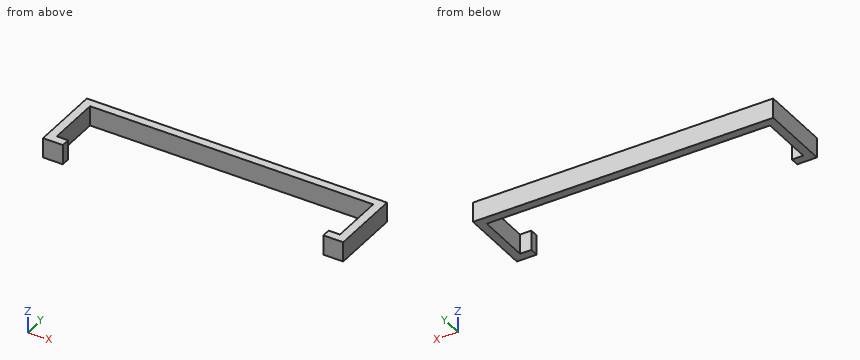
Autodesk Inventor part; units mm, degrees
ref_plane "YZ Plane" through (0, 0, 0) normal (1, 0, 0) x (0, 1, 0)
ref_plane "XZ Plane" through (0, 0, 0) normal (0, 1, 0) x (-1, 0, 0)
ref_plane "XY Plane" through (0, 0, 0) normal (0, 0, 1) x (1, 0, 0)
sketch "Szkic1" plane through (0, 0, 0) normal (0, 1, 0) x (-1, 0, 0)
  point P0 (0, 0)
sketch "Szkic2" plane through (0, 0, 0) normal (0, 1, 0) x (-1, 0, 0)
  line L0 (0, 0) -> (-100, 0)
  line L1 (-100, 0) -> (-100, 7)
  line L2 (-100, 7) -> (0, 7)
  line L3 (0, 7) -> (0, 0)
  dimension "d0" = 100
  dimension "d1" = 7
extrude "Wyciągnięcie proste1" add sketch "Szkic2" along normal blind 3
sketch "Szkic3" plane through (0, 3, 0) normal (0, 1, 0) x (1, 0, 0)
  line L0 (0, 0) -> (-3, 0)
  line L1 (-3, 0) -> (-3, -7)
  line L2 (-3, -7) -> (0, -7)
  line L3 (0, -7) -> (0, 0)
  line L4 (100, -7) -> (100, 0)
  line L5 (100, 0) -> (103, 0)
  line L6 (103, 0) -> (103, -7)
  line L7 (103, -7) -> (100, -7)
  line L8 (100, -7) -> (100, 0)
  dimension "d4" = 3
  dimension "d5" = 7
  dimension "d6" = 3
extrude "Wyciągnięcie proste2" add sketch "Szkic3" against normal blind 22
sketch "Szkic4" plane through (0, -19, 0) normal (0, -1, 0) x (1, 0, 0)
  line L0 (-3, 0) -> (0, 0)
  line L1 (-3, 0) -> (4, 0)
  line L2 (4, 0) -> (4, 7)
  line L3 (4, 7) -> (-3, 7)
  line L4 (-3, 7) -> (-3, 0)
  line L5 (100, 0) -> (103, 0)
  line L6 (103, 0) -> (96, 0)
  line L7 (96, 0) -> (96, 7)
  line L8 (96, 7) -> (103, 7)
  line L9 (103, 7) -> (103, 0)
  dimension "d9" = 7
  dimension "d10" = 7
extrude "Wyciągnięcie proste3" add sketch "Szkic4" along normal blind 3
properties part number "uchwyt"
CAD build for the part. Positions are in the model's coordinates, mm. Round coordinates to 2 decimals unless told otherwise and drop trailing zeros. Order: outer loops, then holes, each group sorted by start corner. A loop starts at its lowest first (then second) coordinate and runs counter-clockwise, first axis right, second up. Notation, with made-up numbers: (19, 85) - (30, 85) arc R33 cw to (30, 116) - close; hole circle Ø10 at (74, 9.5). An arc over 180 degrees is marked (long way). Return JSON: item names as keys, results as strings.
(1) Cut at C-C (x = 77). Give the cut face in (y, z).
Answer key:
{"outline": "(0, 0) - (3, 0) - (3, 7) - (0, 7) - close"}
(2) Pin check, flat tip, straight feed: pin 1 Ø1.5 at (x, z) = (21, 2) entering from -Y. Stop position of the tip, or through.
Answer key:
{"pin 1": "stops at y = 0"}
(3) Cut at A-A (y = -17). Give the cut face in (x, z).
Answer key:
{"outline": "(-3, 0) - (0, 0) - (0, 7) - (-3, 7) - close; (100, 0) - (103, 0) - (103, 7) - (100, 7) - close"}
(4) Cut at B-B (z = 4.5). Give the cut face in (x, y), then the cut area to 3 significant figures.
Answer key:
{"outline": "(-3, -22) - (4, -22) - (4, -19) - (0, -19) - (0, 0) - (100, 0) - (100, -19) - (96, -19) - (96, -22) - (103, -22) - (103, 3) - (-3, 3) - close", "area": "474 mm^2"}
(5) Wall check: probe 1 along X at (y, z) = (-1, 6); probe 2 along Y at (x, z) = (82, 1). Give the ranges that are in metal, low to high. Write a range as from..to.
Answer key:
{"probe 1": "x = -3..0, 100..103", "probe 2": "y = 0..3"}
